```python
from build123d import *

# Parameters (mm, degrees)
F0_R     = 12.7
F1_DEPTH = 139.7
F2_R     = 6.35
F3_DEPTH = 25.4
F5_DEPTH = 2.54
F7_DEPTH = 5.08


with BuildPart() as f1:
    # F0 (on Front) → F1 (new body, symmetric)
    with BuildSketch(Plane.XZ):
        Circle(F0_R)
    extrude(amount=F1_DEPTH, both=True)

    # F2 (on face) → F3 (cut)
    with BuildSketch(Plane.XZ.offset(139.7)):
        Circle(F2_R)
    extrude(amount=-F3_DEPTH, mode=Mode.SUBTRACT)

    # F4 (on face) → F5 (cut)
    with BuildSketch(Plane.XZ.offset(139.7)):
        Polygon((-2.529651, 18.032704), (-2.529651, 12.445516), (-2.529651, -12.445516), (-2.529651, -16.867724), (2.550349, -16.867724), (2.550349, -12.441291), (2.550349, 12.445516), (2.550349, 18.032704), align=None)
    extrude(amount=-F5_DEPTH, mode=Mode.SUBTRACT)

    # F6 (on face) → F7 (cut)
    with BuildSketch(Plane.XZ.offset(139.7)):
        Polygon((25.367279, -2.379521), (25.367279, 0), (25.367279, 2.700479), (-15.440687, 2.700479), (-15.440687, -2.379521), align=None)
    extrude(amount=-F7_DEPTH, mode=Mode.SUBTRACT)


solid = f1.part
```
Input: part model. Units: mm. Frame: model coordinates. A direction names the side the tool comes from. Give positions to 0.01 mm unless a question says otherwise; leave off trailing zeros. Write each loop counter-clockwise with the first axis right and the second up, starting at its lowest first coordinate (ties: lowest second). Pieces come first, ordered by that corner, then holes. Notation, with made-up numbers: (-31, 37) - (1, 37) arc R23 cw to (1, 64) - close; hole circle Ø7 at (34, 20). An arc over 180 degrees is marked (long way). Write item = value, one per line. Start each with the question number.
1. Mould query, pull axis X, two halves, no side actions, for faces 1 (the flat face through (0, -137.16, -9)), 2 (the flat face through (-6, -139.7, -6)), 3 (the cylindrical face through (-2.75, -1.96, -12.4)). Classes: released by +X, released by -X, zero draft, split by the parting line, or undercut.
2. Section query B-B, the plane y = 11.5. Output: boundary loops of the cut face in (x, z), then the cut area to 3 significant figures.
3. Ray query, L1, parallel to Z at x = 0, y = -119.75; L2, parallel to Y at x = 7.25, z = 0.75. Return the intervals inside material, ascending.
4. Section query C-C, the plane x = -10. Output: boundary loops of the cut face in (y, z), then the cut area to 3 significant figures.
5. Section query A-A, the plane x = 0. Output: boundary loops of the cut face in (y, z), then the cut area to 3 significant figures.
6. Access query for faces 4 (the flat face through (0, -114.3, 0)), 5 (the flat face through (0, -137.16, 9)), 6 (the flat face through (0, 139.7, 0)), 7 (the flat face through (-9, -134.62, 0)). Directions: +Z, -Z, +X, -X, +Y, -Y. A direction counts if a zero-diameter tool reaches every point of the face in a straight line with its end or side. Return the directions, or none.
7. First-contact query: pin 1 Ø5 at (x, y) = (9.5, 79.5) entering from +Z; pin 2 Ø7.5 at (x, z) = (0, 0) entering from -Y; pin 3 Ø1.5 at (x, z) = (1, 8) entering from -Y. Flat tips, straight axial feed; report the tip coordinate or a pass-through.
Check sheet entries:
q1.face_1 = undercut
q1.face_2 = zero draft
q1.face_3 = split by the parting line
q2.outline = circle Ø25.4 at (0, 0)
q2.area = 507 mm2
q3.L1 = -12.7 to -6.35, 6.35 to 12.7
q3.L2 = -134.62 to 139.7
q4.outline = (-139.7, -7.83) - (139.7, -7.83) - (139.7, 7.83) - (-139.7, 7.83) - (-139.7, 2.7) - (-134.62, 2.7) - (-134.62, -2.38) - (-139.7, -2.38) - close
q4.area = 4,350 mm2
q5.outline = (-137.16, -12.7) - (139.7, -12.7) - (139.7, 12.7) - (-137.16, 12.7) - (-137.16, 6.35) - (-114.3, 6.35) - (-114.3, -6.35) - (-137.16, -6.35) - close
q5.area = 6,740 mm2
q6.face_4 = -Y
q6.face_5 = +Z, -Z, -Y
q6.face_6 = +Z, -Z, +X, -X, +Y
q6.face_7 = +X, -X, -Y
q7.pin_1 = 10.6
q7.pin_2 = -114.3
q7.pin_3 = -137.16
